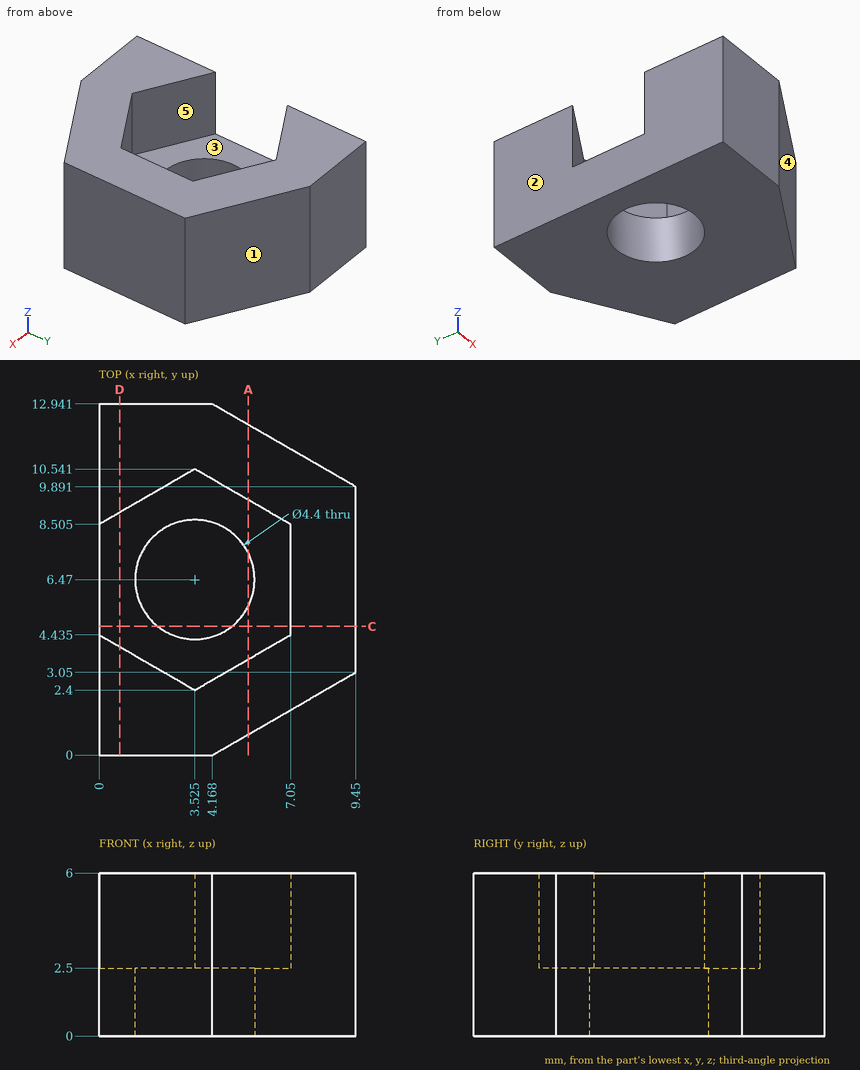
Part print with two shaded views. Sizes in mm from the minimum x, y, z corner. A direction names the side the tool comes from. Give positions to 0.01 mm unless a question says otherwise; leave off trailing zeros. Write each loop counter-clockwise with the first axis right and the second up, starting at its lowest first coordinate (ties: lowest second). Pieces come first, ordered by that corner, then holes.
1) Probe L1, parallel to X at y = 5, z = 5; L2, parallel to Z at x = 1.75, y = 4; L3, parallel to Y at x = 4.5, z = 2.8. List the from-to ranges inside material, lowest first.
Resolved:
L1: x = 7.05 to 9.45
L2: z = 0 to 2.5
L3: y = 0.19 to 2.96, 9.98 to 12.75
2) Cut at C-C on y = 4.75. Write the cut outline in (x, z).
Resolved:
outline: (0, 0) - (2.15, 0) - (2.15, 2.5) - (0, 2.5) - close; (4.9, 0) - (9.45, 0) - (9.45, 6) - (7.05, 6) - (7.05, 2.5) - (4.9, 2.5) - close
3) Two-plate mould, pull along Y, no slides. Class the marked faces 1, 2 and 3: released by +Y, released by -Y, zero draft, split by the parting line, or undercut.
Resolved:
face 1: released by +Y
face 2: zero draft
face 3: undercut
4) Which spindle directions (+Z, -Z, +X, -X, +Y, -Y) get a long thin tool onto all of the face, cutting with end or side? Do the marked faces 4 and 5. Say none if no direction does.
Resolved:
face 4: +Z, -Z, +X, -Y
face 5: +Z
5) Cut at D-D on x = 0.75. Write the cut outline in (y, z).
Resolved:
outline: (0, 0) - (12.94, 0) - (12.94, 6) - (8.94, 6) - (8.94, 2.5) - (4, 2.5) - (4, 6) - (0, 6) - close
6) Cut at A-A on x = 5.5. Write the cut outline in (y, z).
Resolved:
outline: (0.77, 0) - (5.5, 0) - (5.5, 2.5) - (3.54, 2.5) - (3.54, 6) - (0.77, 6) - close; (7.44, 0) - (12.17, 0) - (12.17, 6) - (9.4, 6) - (9.4, 2.5) - (7.44, 2.5) - close
7) Pin check, flat tips, straight feed: pin 1 (1 mm diameter, centred on y = 6, z = 5, fed in from -X); pin 2 (1.5 mm diameter, centred on x = 6, z = 3, fed in from +Y) (1 decimal). Stop position of each tip, or through.
Resolved:
pin 1: stops at x = 7.05
pin 2: stops at y = 12.3
